For this review, take the finished solid that the model builds, in its own axes (mm). Face numbers are marked on the shaded views. A direction names the side the tool comes from. Coordinates: 2 decimals unless noted, no trailing zeros. Loops run counter-clockwise (first coordinate to the right, second up) from the corner with the lowest first, then second, coordinate; pieces in that order, holes last. Notation, with made-up numbers: M -13,6.25 L 40,6.25 A22 cw 40,26.25 Z; hole C 55.25,-21 d11. An arc over 180 degrees is marked long. Put each result on its own line as item: value.
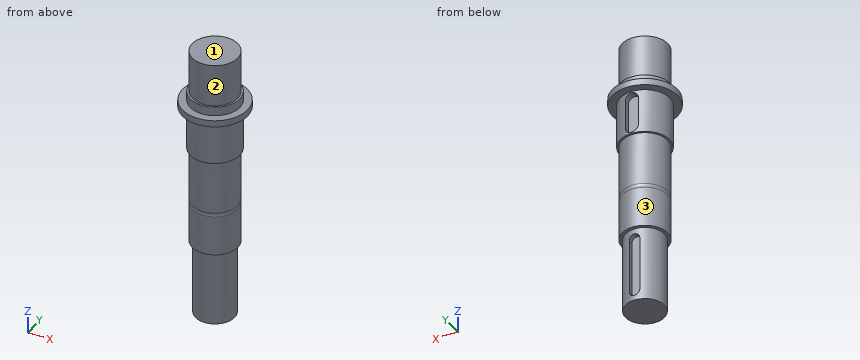
```python
from build123d import *

# Parameters (mm, degrees)
CUT_EXTRUDE1_REACH      = 219.22
CUT_EXTRUDE1_END_RADIUS = 19
CUT_EXTRUDE2_REACH      = 218.701
CUT_EXTRUDE2_END_RADIUS = 15


with BuildPart() as part:
    # Sketch1 → Revolve1 (revolve)
    with BuildSketch(Plane(origin=(0, 0, 0), x_dir=(0, 0, -1), z_dir=(1, 0, 0))):
        with BuildLine():
            Line((0, 0), (0, 15))
            Line((0, 15), (-58, 15))
            Line((-58, 15), (-58, 17.5))
            Line((-58, 17.5), (-89, 17.5))
            ThreePointArc((-89, 17.5), (-90.5612495, 17.25), (-92.122498999, 17.5))
            Line((-92.122498999, 17.5), (-133.472498999, 17.5))
            Line((-133.472498999, 17.5), (-133.472498999, 19))
            Line((-133.472498999, 19), (-167.472498999, 19))
            Line((-167.472498999, 19), (-167.472498999, 25))
            Line((-167.472498999, 25), (-172.472498999, 25))
            Line((-172.472498999, 25), (-172.472498999, 19))
            Line((-172.472498999, 19), (-179.472498999, 19))
            Line((-179.472498999, 19), (-179.472498999, 17.5))
            Line((-179.472498999, 17.5), (-212.222498999, 17.5))
            Line((-212.222498999, 17.5), (-212.222498999, 0))
            Line((-212.222498999, 0), (0, 0))
        make_face()
    revolve(axis=Axis((0, 0, 0), (0, 0, 1)))

    # Cut-Extrude1: up to this cylinder (the profile starts inside it)
    cut_extrude1_end = Plane(origin=(0, 0, 150.472499), z_dir=(0, 0, -1)) * Cylinder(CUT_EXTRUDE1_END_RADIUS, 477.44, mode=Mode.PRIVATE)
    # Sketch2 → Cut-Extrude1 (cut, up to the surface)
    with BuildSketch(Plane(origin=(0, 14, 0), x_dir=(1, 0, 0), z_dir=(0, 1, 0)), mode=Mode.PRIVATE) as cut_extrude1_sk1:
        with BuildLine():
            Line((5, -139.472498999), (5, -161.472498999))
            ThreePointArc((5, -161.472498999), (0, -166.472498999), (-5, -161.472498999))
            Line((-5, -161.472498999), (-5, -139.472498999))
            ThreePointArc((-5, -139.472498999), (0, -134.472498999), (5, -139.472498999))
        make_face()
    cut_extrude1_tool1 = extrude(cut_extrude1_sk1.sketch, amount=CUT_EXTRUDE1_REACH, mode=Mode.PRIVATE) & cut_extrude1_end
    add(cut_extrude1_tool1.solids().sort_by_distance((0, 14, 150.472499))[0], mode=Mode.SUBTRACT)

    # Cut-Extrude2: up to this cylinder (the profile starts inside it)
    cut_extrude2_end = Plane(origin=(0, 0, 29), z_dir=(0, 0, -1)) * Cylinder(CUT_EXTRUDE2_END_RADIUS, 468.402, mode=Mode.PRIVATE)
    # Sketch3 → Cut-Extrude2 (cut, up to the surface)
    with BuildSketch(Plane(origin=(0, 11, 0), x_dir=(1, 0, 0), z_dir=(0, 1, 0)), mode=Mode.PRIVATE) as cut_extrude2_sk1:
        with BuildLine():
            Line((-4, -50), (-4, -8))
            ThreePointArc((-4, -8), (0, -4), (4, -8))
            Line((4, -8), (4, -50))
            ThreePointArc((4, -50), (0, -54), (-4, -50))
        make_face()
    cut_extrude2_tool1 = extrude(cut_extrude2_sk1.sketch, amount=CUT_EXTRUDE2_REACH, mode=Mode.PRIVATE) & cut_extrude2_end
    add(cut_extrude2_tool1.solids().sort_by_distance((0, 11, 29))[0], mode=Mode.SUBTRACT)


solid = part.part
```
(1) Add section B-B (z = 108). Write out the cut boundary in (x, y), plus the area to 3 significant figures.
Determined:
outline: C 0,0 d35
area: 962 mm^2
(2) Add section A-A (y = 0). Write out the cut boundary in (x, z).
Determined:
outline: M -25,167.47 L -19,167.47 L -19,133.47 L -17.5,133.47 L -17.5,92.12 A5 cw -17.5,89 L -17.5,58 L -15,58 L -15,0 L 15,0 L 15,58 L 17.5,58 L 17.5,89 A5 cw 17.5,92.12 L 17.5,133.47 L 19,133.47 L 19,167.47 L 25,167.47 L 25,172.47 L 19,172.47 L 19,179.47 L 17.5,179.47 L 17.5,212.22 L -17.5,212.22 L -17.5,179.47 L -19,179.47 L -19,172.47 L -25,172.47 Z
(3) Wall thickness on line 1 along Z through (x, y) = (0, 13.5); line 2 along X through (y, z) = (13.5, 25.5); line 3 along Z through (x, y) = (2, 21): over which ranges is each line inside the solid? List them lowest first. Write a range as [from, to].
Determined:
line 1: z = [0, 4], [54, 212.22]
line 2: x = [-6.54, -4], [4, 6.54]
line 3: z = [167.47, 172.47]
(4) For pin 1 (3 mm diameter, centred on x = 1.5, z = 153.5, fed in from +Y); pin 2 (2 mm diameter, centred on y = 0.5, z = 115.5, fed in from +X); pin 3 (5 mm diameter, centred on y = 17, z = 156, fed in from +X), all flat-tipped, find the tip position at first contact; note any pin that passes through.
Determined:
pin 1: stops at y = 14
pin 2: stops at x = 17.5
pin 3: stops at x = 12.28
(5) Add section C-C (x = -21). Write out the cut boundary in (y, z), plus the area to 3 significant figures.
Determined:
outline: M -13.56,167.47 L 13.56,167.47 L 13.56,172.47 L -13.56,172.47 Z
area: 136 mm^2
(6) Tool access review of the marked faces 1, 2 and 3: name each direction out of +Z, -Z, +X, -X, +Y, -Y from which nothing blocks a thin tool from reaching the whole face with its end or side.
Determined:
face 1: +Z, +X, -X, +Y, -Y
face 2: +Z
face 3: -Z
(7) Add section D-D (y = -22). Write out the cut boundary in (x, z), plus the area to 3 significant figures.
Determined:
outline: M -11.87,167.47 L 11.87,167.47 L 11.87,172.47 L -11.87,172.47 Z
area: 119 mm^2
